```python
from build123d import *

# Parameters (mm, degrees)
SKETCH1_R           = 0.5
BOSS_EXTRUDE1_DEPTH = 3


with BuildPart() as part:
    # Sketch1 → Boss-Extrude1 (new body)
    with BuildSketch(Plane(origin=(0, 0, 0), x_dir=(1, 0, 0), z_dir=(0, 1, 0))):
        Polygon((42.8625, 26.9875), (42.8625, 30.3375), (39.8625, 30.3375), (39.8625, 36.6875), (42.8625, 36.6875), (42.8625, 39.6875), (7.9375, 39.6875), (7.9375, 36.6875), (-17.4625, 36.6875), (-17.4625, 39.6875), (-30.1625, 39.6875), (-30.1625, 36.6875), (-55.5625, 36.6875), (-55.5625, 39.6875), (-68.2625, 39.6875), (-68.2625, 33.6875), (-65.2625, 33.6875), (-65.2625, 8.2875), (-68.2625, 8.2875), (-68.2625, -8.2875), (-65.2625, -8.2875), (-65.2625, -33.6875), (-68.2625, -33.6875), (-68.2625, -39.6875), (-55.5625, -39.6875), (-55.5625, -36.6875), (-30.1625, -36.6875), (-30.1625, -39.6875), (-17.4625, -39.6875), (-17.4625, -36.6875), (7.9375, -36.6875), (7.9375, -39.6875), (42.8625, -39.6875), (42.8625, -36.6875), (39.8625, -36.6875), (39.8625, -30.3375), (42.8625, -30.3375), (42.8625, -26.9875), (-42.8625, -26.9875), (-42.8625, 26.9875), align=None)
        with Locations(Location((-44.361566376, 28.486566376, 0), (0, 0, 270))):
            Circle(SKETCH1_R, mode=Mode.SUBTRACT)
        with Locations(Location((-44.361566376, -28.486566376, 0), (0, 0, 270))):
            Circle(SKETCH1_R, mode=Mode.SUBTRACT)
    extrude(amount=BOSS_EXTRUDE1_DEPTH)


solid = part.part
```
Input: part model. Units: mm. Frame: model coordinates. A direction names the side the tool comes from. Coordinates: 2 decimals unless noted, no trailing zeros. Loops run counter-clockwise (first coordinate to the right, second up) from the corner with the lowest first, then second, coordinate; pieces in that order, holes last. Notation, with made-up numbers: (-5, 49) - (51, 49) arc R20 ccw to (51, 55) - close; hole circle Ø5 at (-3, 56). An arc over 180 degrees is marked (long way). Answer in a Markdown table with one row per item.
(1) Cut plane C-C on y = 1.15. Count the separate pieces of the cut face and the enclosed holes in it, plus the area to 3 significant figures.
Model answer:
| item | result |
|---|---|
| separate pieces | 1 |
| enclosed holes | 2 |
| area | 3,700 mm² |
(2) Cut plane A-A on x = -0.5. Output: boundary loops of the cut face in (y, z).
Model answer:
| item | result |
|---|---|
| outline | (0, -36.69) - (3, -36.69) - (3, -26.99) - (0, -26.99) - close; (0, 26.99) - (3, 26.99) - (3, 36.69) - (0, 36.69) - close |
(3) Cut plane B-B on z = -14. Output: boundary loops of the cut face in (x, y), plus the area to 3 significant figures.
Model answer:
| item | result |
|---|---|
| outline | (-65.26, 0) - (-42.86, 0) - (-42.86, 3) - (-65.26, 3) - close |
| area | 67.2 mm² |
(4) Material intervals for L1, parallel to Z at x = -24, y = 2.5; L2, parallel to Z at x = -9, y = 2.8; L3, parallel to X at y = 2, z = 31, sorted ascending. Write a range as from..to.
Model answer:
| item | result |
|---|---|
| L1 | z = -39.69..-26.99, 26.99..39.69 |
| L2 | z = -36.69..-26.99, 26.99..36.69 |
| L3 | x = -65.26..39.86 |
(5) Mould query, pull axis Z, two halves, no side actions, for faces 5 (the face through (-43, 1, -36.688)), 6 (the face through (-62, 1, 39.688)), 7 (the face through (39.862, 1, 34)). Classes: pulls with the +Z half, pulls with the -Z half, needs draft (parallel to the pull), parting line crosses it, or undercut.
Model answer:
| item | result |
|---|---|
| face 5 | pulls with the -Z half |
| face 6 | pulls with the +Z half |
| face 7 | undercut |
(6) Set-up query: faces 1 (the face through (-17.462, 1, 38)), 2 (the face through (-55.562, 1, -38)), 3 (the face through (41, 1, -30.338)), 4 (the face through (-67, 1, -33.688)). Return all of +Z, -Z, +X, -X, +Y, -Y with unobstructed straight access to the full face (end or side cutting, diameter ignored); none if empty.
Model answer:
| item | result |
|---|---|
| face 1 | +Z, +Y, -Y |
| face 2 | -Z, +Y, -Y |
| face 3 | +X, +Y, -Y |
| face 4 | -X, +Y, -Y |
(7) Cut plane D-D on x = -54. Output: boundary loops of the cut face in (y, z), plus the area to 3 significant figures.
Model answer:
| item | result |
|---|---|
| outline | (0, -36.69) - (3, -36.69) - (3, 36.69) - (0, 36.69) - close |
| area | 220 mm² |
(8) Pin query (flat end, axial travel): P1, Ø1.5, axis at x = -6, y = 1.5, coming from the -Z side; P2, Ø1.5, axis at x = -2, y = 1, coming from the +Z side. Return the tip coordinate at first contact, or that it passes through.
Model answer:
| item | result |
|---|---|
| P1 | stops at z = -36.69 |
| P2 | stops at z = 36.69 |
